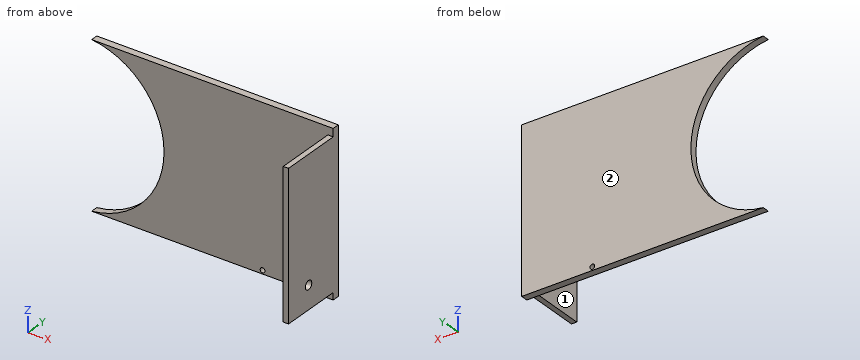
Autodesk Inventor part; units mm, degrees
ref_plane "YZ Plane" through (0, 0, 0) normal (1, 0, 0) x (0, 1, 0)
ref_plane "XZ Plane" through (0, 0, 0) normal (0, 1, 0) x (-1, 0, 0)
ref_plane "XY Plane" through (0, 0, 0) normal (0, 0, 1) x (1, 0, 0)
sketch "Esboço1" plane through (0, 0, 0) normal (0, 1, 0) x (-1, 0, 0)
  line L0 (-70.7559, -45.75) -> (70.7559, -45.75)
  line L1 (70.7559, 45.75) -> (-70.7559, 45.75)
  line L2 (-70.7559, 45.75) -> (-70.7559, -45.75)
  line L3 (-70.7559, -45.75) -> (70.7559, 45.75) construction
  line L4 (70.7559, -45.75) -> (-70.7559, 45.75) construction
  arc A0 (66.0067, 45.75) -> (66.0067, -45.75) centre (71.083, 0) ccw
  circle A1 centre (-30.7559, -43.75) radius 1.35
  point P0 (0, 0)
  dimension "d3" = 2.7
  dimension "d4" = 2
  dimension "d5" = 40
  dimension "d15" = 91.5
extrude "Extrusão1" add sketch "Esboço1" along normal blind 4
sketch "Esboço2" plane through (0, 0, 0) normal (0, -1, 0) x (1, 0, 0)
  line L0 (-66.0067, 45.75) -> (70.7559, 45.75)
  line L1 (70.7559, -45.75) -> (-66.0067, -45.75)
  line L2 (70.7559, 45.75) -> (67.7559, 45.75)
  line L3 (67.7559, 45.75) -> (67.7559, -45.75)
  line L4 (67.7559, -45.75) -> (70.7559, -45.75)
  line L5 (70.7559, -45.75) -> (70.7559, 45.75)
  line L6 (67.7559, -41.75) -> (70.7559, -41.75)
  line L7 (70.7559, -41.75) -> (70.7559, 41.25)
  line L8 (70.7559, 41.25) -> (67.7559, 41.25)
  line L9 (67.7559, 41.25) -> (67.7559, -41.75)
  line L10 (67.7559, -41.75) -> (70.7559, 41.25) construction
  line L11 (70.7559, -41.75) -> (67.7559, 41.25) construction
  point P0 (0, 0)
  point P1 (69.2559, -0.25)
  point P2 (70.7559, 41.25)
  point P3 (67.7559, 41.25)
  point P4 (67.7559, -41.75)
  point P5 (70.7559, -41.75)
  point P6 (69.2559, -41.75)
  point P7 (69.2559, -45.75)
  point P8 (69.2559, 45.75)
  point P9 (69.2559, 41.25)
  dimension "d8" = 3
  dimension "d9" = 3
  dimension "d10" = 83
  dimension "d14" = 4.5
extrude "Extrusão2" add sketch "Esboço2" along normal blind 35 contours L8 L5 L6 L3
sketch "Esboço3" plane through (70.7559, 0, -45.75) normal (1, 0, 0) x (0, 0, -1)
  circle A0 centre (-17.2006, -19.299) radius 2.5
  point P0 (-45.75, 0)
  dimension "d16" = 5
hole "Furo1" at (70.7559, -19.299, -28.5494) direction (-1, 0, 0) diameter 5 end through all
properties part number "TAMPA_BASE"
Input: part model. Units: mm. Frame: model coordinates. Face numbers are marked on the shaded views. A direction names the side the tool comes from. Round coordinates to 2 decimals unless told otherwise and drop trailing zeros. Loops run counter-clockwise (first coordinate to the right, second up) from the corner with the lowest first, then second, coordinate; pieces in that order, holes last. Notation, with made-up numbers: M -28.75,29 L 17.25,29 A18 cw 17.25,60 Z; hole C 34.5,-28.75 d1. An arc over 180 degrees is marked long. Answer in a Markdown table with one row per item. Add a question column.
1. Section D-D (y = -11.5). Output: boundary loops of the cut face in (x, z), and give its area (3 significant figures).
2. Section B-B (x = 22.5). Output: boundary loops of the cut face in (y, z), and give its area (3 significant figures).
3. Set-up query: the marked faces 1 and 2. Return all of +Z, -Z, +X, -X, +Y, -Y with unobstructed straight access to the full face (end or side cutting, diameter ignored); none if empty.
4. Section C-C (z = 14). Output: boundary loops of the cut face in (x, y), and give its area (3 significant figures).
5. Contact query for flat-ended pins moving along their axis: pin 1 (8 mm diameter, centred on x = -10, y = -5, fed in from +Z); pin 2 (3.5 mm diameter, centred on x = 69, y = -12, fed in from -Z); pin 3 (2.5 mm diameter, centred on x = 69, y = -14, fed in from +Z); pin 4 (6 mm diameter, centred on y = -19.3, z = -28.55, fed in from +X). Output: stop coordinate, or through.
6. Section A-A (x = -48.5). Output: boundary loops of the cut face in (y, z).
7. Ray query, probe 1 along Y at (x, z) = (29.5, -1); probe 2 along X at (y, z) = (-1, -34.5). Return the intervals inside material, ascending.
Values follow:
| question | item | result |
|---|---|---|
| 1 | outline | M 67.76,-41.75 L 70.76,-41.75 L 70.76,41.25 L 67.76,41.25 Z |
| 1 | area | 249 mm^2 |
| 2 | outline | M 0,-45.75 L 4,-45.75 L 4,45.75 L 0,45.75 Z |
| 2 | area | 366 mm^2 |
| 3 | face 1 | +Z, -Z, -X, -Y |
| 3 | face 2 | +Z, -Z, +X, -X, +Y |
| 4 | outline | M -27.23,0 L 67.76,0 L 67.76,-35 L 70.76,-35 L 70.76,4 L -27.23,4 Z |
| 4 | area | 497 mm^2 |
| 5 | pin 1 | through |
| 5 | pin 2 | z = -41.75 |
| 5 | pin 3 | z = 41.25 |
| 5 | pin 4 | x = 70.76 |
| 6 | outline | M 0,-45.75 L 4,-45.75 L 4,-40.11 L 0,-40.11 Z; M 0,40.11 L 4,40.11 L 4,45.75 L 0,45.75 Z |
| 7 | probe 1 | 0 to 4 |
| 7 | probe 2 | 67.76 to 70.76 |
